Input: part model. Units: mm. Frame: model coordinates. A direction names the side the tool comes from. Give positions to 0.01 mm unless a question says otherwise; leave off trailing zeros. Loops run counter-clockwise (first coordinate to the right, second up) from the corner with the lowest first, then second, coordinate; pieces in that order, holes last. Notation, with made-up numbers: M 56.5,68 L 60.5,68 A8 cw 60.5,78 Z; hole C 85,-32.5 d4. An arc over 180 degrees is marked long. Answer as a JSON object with one key per item and string values. Group by question number.
1) First-contact query: P1, Ø1, axis at x = -16.5, y = -65, coming from the -Z side; P2, Ø0.9, axis at x = 29.5, z = 1, coming from the +Y side. Flat tips, straight axial feed; report the tip coordinate or a pass-through.
2) Ray query, L1, parallel to X at y = -53, z = 0.8; L2, parallel to Y at x = 6.5, z = 2.4; L3, parallel to Y at x = 6, z = 1. Return the intervals inside material, ascending.
3) Draft query along X for faces 3 (the cylindrical face through (-0.38, -67.71, 1.52)), 4 (the flat face through (-35, -18, 1)), 5 (the flat face through (0, 30, 1)). Return one class per face: +X half, -X half, draft (parallel to the pull), parting line (faces both ways), or undercut.
4) Section query A-A on z = 1.55. Count the separate pieces of the cut face and the enclosed holes in it, plus the area to 3 significant figures.
5) Access query for faces 1 (the flat face through (2.5, -20, 1)), 2 (the flat face through (-7, -22, 3)). Directions: +Z, -Z, +X, -X, +Y, -Y. A direction counts if a zero-diameter tool reaches every point of the face in a straight line with its end or side. Return the directions, or none.
6) Section query C-C on x = -19. Return loops of the section in (y, z), plus the area to 3 significant figures.
7) Section query B-B on x = 13. Return loops of the section in (y, z).
from build123d import *

# Parameters (mm, degrees)
SKETCH1_R           = 2.5
BOSS_EXTRUDE1_DEPTH = 3
FILLET1_R           = 10
FILLET1_R_2         = 15
FILLET1_R_3         = 50
SKETCH2_R           = 1.75
SKETCH2_R_2         = 12
CUT_EXTRUDE1_DEPTH  = 84.903310475
SKETCH4_W           = 3
SKETCH4_H           = 16
CUT_EXTRUDE3_DEPTH  = 84.903310475
SKETCH9_R           = 1.5
CUT_EXTRUDE4_DEPTH  = 84.903310475


with BuildPart() as part:
    # Sketch1 → Boss-Extrude1 (new body)
    with BuildSketch(Plane.XY):
        Polygon((-35, 30), (35, 30), (35, -62.640754554), (0, -87.640754554), (-35, -62.640754554), align=None)
        with Locations((25, 20)):
            Circle(SKETCH1_R, mode=Mode.SUBTRACT)
        with Locations((-25, 20)):
            Circle(SKETCH1_R, mode=Mode.SUBTRACT)
        with BuildLine():
            Line((2.5, -16.5), (2.5, -23.5))
            ThreePointArc((2.5, -23.5), (0, -26), (-2.5, -23.5))
            Line((-2.5, -23.5), (-2.5, -16.5))
            ThreePointArc((-2.5, -16.5), (0, -14), (2.5, -16.5))
        make_face(mode=Mode.SUBTRACT)
    extrude(amount=BOSS_EXTRUDE1_DEPTH)

    # Fillet1
    # the kernel refuses this fillet: 50, 15, 10 mm, written as the material it takes off along each edge
    with BuildSketch(Plane(origin=(35, 30, -25), x_dir=(-1, 0, 0), z_dir=(0, 0, 1))) as fillet1_piece_1:
        with BuildLine():
            CenterArc((FILLET1_R, FILLET1_R), FILLET1_R, 180, 90)
            Line((0, FILLET1_R), (0, 0))
            Line((0, 0), (FILLET1_R, 0))
        make_face()
    extrude(amount=53, mode=Mode.SUBTRACT)
    with BuildSketch(Plane(origin=(-35, 30, -25), x_dir=(1, 0, 0), z_dir=(0, 0, 1))) as fillet1_piece_2:
        with BuildLine():
            CenterArc((FILLET1_R, -FILLET1_R), FILLET1_R, 90, 90)
            Line((0, -FILLET1_R), (0, 0))
            Line((0, 0), (FILLET1_R, 0))
        make_face()
    extrude(amount=53, mode=Mode.SUBTRACT)
    with BuildSketch(Plane(origin=(-35, -62.640754554, -19.298171073), x_dir=(0.8137334712067342, -0.5812381937190976, 0), z_dir=(0, 0, 1)), Plane(origin=(35, -62.640754554, -19.298171073), x_dir=(0, 1, 0), z_dir=(0, 0, 1))) as fillet1_piece_3:
        with BuildLine():
            CenterArc((FILLET1_R_2 * 0.514617895292, FILLET1_R_2), FILLET1_R_2, 215.537677792, 54.462322208)
            Line((-FILLET1_R_2 * 0.299115575915, FILLET1_R_2 * 0.418761806281), (0, 0))
            Line((0, 0), (FILLET1_R_2 * 0.514617895292, 0))
        make_face()
    extrude(amount=41.596342147, mode=Mode.SUBTRACT)
    with BuildSketch(Plane(origin=(0, -87.640754554, -89.285714286), x_dir=(0.8137334712067352, 0.5812381937190962, 0), z_dir=(0, 0, 1))) as fillet1_piece_4:
        with BuildLine():
            CenterArc((FILLET1_R_3 * 0.714285714286, FILLET1_R_3), FILLET1_R_3, 198.924644416, 71.075355584)
            Line((-FILLET1_R_3 * 0.23166023166, FILLET1_R_3 * 0.675675675676), (0, 0))
            Line((0, 0), (FILLET1_R_3 * 0.714285714286, 0))
        make_face()
    extrude(amount=181.571428571, mode=Mode.SUBTRACT)

    # Sketch2 → Cut-Extrude1 (cut, through all)
    with BuildSketch(Plane.XY.offset(3)):
        with Locations((24, -42)):
            Circle(SKETCH2_R)
        with Locations((0, -42)):
            Circle(SKETCH2_R)
        with Locations((0, -66)):
            Circle(SKETCH2_R)
        with Locations((24, -66)):
            Circle(SKETCH2_R)
        with Locations((12, -54)):
            Circle(SKETCH2_R_2)
    extrude(amount=-CUT_EXTRUDE1_DEPTH, mode=Mode.SUBTRACT)

    # Sketch4 → Cut-Extrude3 (cut, through all)
    with BuildSketch(Plane.XY.offset(3)):
        with Locations((29, -21)):
            Rectangle(SKETCH4_W, SKETCH4_H)
        with Locations((-29, -21)):
            Rectangle(SKETCH4_W, SKETCH4_H)
    extrude(amount=-CUT_EXTRUDE3_DEPTH, mode=Mode.SUBTRACT)

    # Sketch9 → Cut-Extrude4 (cut, through all)
    with BuildSketch(Plane.XY.offset(3)):
        with Locations((-27.875, -54)):
            Circle(SKETCH9_R)
        with Locations((-9.125, -54)):
            Circle(SKETCH9_R)
    extrude(amount=-CUT_EXTRUDE4_DEPTH, mode=Mode.SUBTRACT)


solid = part.part
Output:
{
 "1": {"P1": "stops at z = 0", "P2": "stops at y = 29.14"},
 "2": {"L1": "x = -35 to -28.99, -26.76 to -10.24, -8.01 to 0.04, 23.96 to 35", "L2": "y = -75.77 to -64.67, -43.33 to 30", "L3": "y = -75.83 to -64.39, -43.61 to 30"},
 "3": {"face 3": "undercut", "face 4": "-X half", "face 5": "draft"},
 "4": {"separate pieces": "1", "enclosed holes": "12", "area": "6,370 mm^2"},
 "5": {"face 1": "+Z, -Z", "face 2": "+Z, +X, -X, +Y, -Y"},
 "6": {"outline": "M -72.44,0 L 30,0 L 30,3 L -72.44,3 Z", "area": "307 mm^2"},
 "7": {"outline": "M -74.48,0 L -65.96,0 L -65.96,3 L -74.48,3 Z; M -42.04,0 L 30,0 L 30,3 L -42.04,3 Z"}
}
